```python
from build123d import *

# Parameters (mm, degrees)
SKETCH1_W           = 35
SKETCH1_H           = 30
BOSS_EXTRUDE5_DEPTH = 2
BOSS_EXTRUDE6_DEPTH = 1


with BuildPart() as part:
    # Sketch1 → Boss-Extrude5 (new body)
    with BuildSketch(Plane.XY):
        with Locations((0, -15)):
            Rectangle(SKETCH1_W, SKETCH1_H)
    extrude(amount=BOSS_EXTRUDE5_DEPTH)

    # Sketch1<7> → Boss-Extrude6 (add)
    with BuildSketch(Plane.XY):
        Polygon((-12.5, 10), (-12.5, 30), (-17.5, 30), (-17.5, 10), (-17.5, 0), (17.5, 0), (17.5, 10), (17.5, 30), (12.5, 30), (12.5, 10), (7.5, 10), (7.5, 30), (2.5, 30), (2.5, 10), (-2.5, 10), (-2.5, 30), (-7.5, 30), (-7.5, 10), align=None)
    extrude(amount=BOSS_EXTRUDE6_DEPTH)


solid = part.part
```
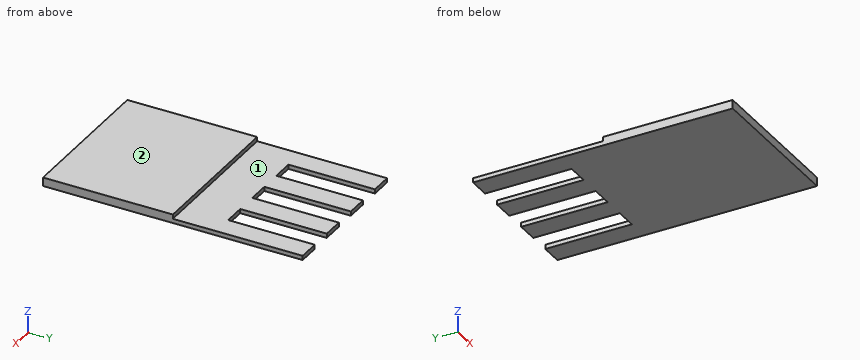
Verification items for the finished model (mm, model axes). Face numbers are marked on the shaded views. A direction names the side the tool comes from. Coordinates: 2 decimals unless noted, no trailing zeros. Loops run counter-clockwise (first coordinate to the right, second up) from the corner with the lowest first, then second, coordinate; pieces in that order, holes last. Notation, with made-up numbers: (-33.75, 79.25) - (-0.75, 79.25) arc R28 cw to (-0.75, 110.25) - close; hole circle Ø6 at (-35, 29.5). An arc over 180 degrees is marked (long way). Put each result on its own line as item: value.
Item 1: Section check C-C (z = 0.3). Enter the section's corners in (x, y).
Conclusion:
outline: (-17.5, -30) - (17.5, -30) - (17.5, 30) - (12.5, 30) - (12.5, 10) - (7.5, 10) - (7.5, 30) - (2.5, 30) - (2.5, 10) - (-2.5, 10) - (-2.5, 30) - (-7.5, 30) - (-7.5, 10) - (-12.5, 10) - (-12.5, 30) - (-17.5, 30) - close
Item 2: Gauge pin test, flat ends, axial feed: pin 1 Ø1 at (x, y) = (13.5, 2) entering from +Z; pin 2 Ø1.1 at (x, z) = (11, 0.5) entering from +Y. Record the tip position at first contact, or that the pin passes through.
Conclusion:
pin 1: stops at z = 1
pin 2: stops at y = 10
Item 3: Section check A-A (y = 21). Enter the section's corners in (x, z).
Conclusion:
outline: (-17.5, 0) - (-12.5, 0) - (-12.5, 1) - (-17.5, 1) - close; (-7.5, 0) - (-2.5, 0) - (-2.5, 1) - (-7.5, 1) - close; (2.5, 0) - (7.5, 0) - (7.5, 1) - (2.5, 1) - close; (12.5, 0) - (17.5, 0) - (17.5, 1) - (12.5, 1) - close
Item 4: Section check B-B (x = -11.5). Enter the section's corners in (y, z).
Conclusion:
outline: (-30, 0) - (10, 0) - (10, 1) - (0, 1) - (0, 2) - (-30, 2) - close
Item 5: Scan lines: line 1 along X through (y, z) = (19, 0.85); line 2 along Y through (x, z) = (-15.5, 1.65); line 3 along Z through (x, y) = (-1, 2.5). Record each from-to range of solid material in increasing order.
Conclusion:
line 1: x = -17.5 to -12.5, -7.5 to -2.5, 2.5 to 7.5, 12.5 to 17.5
line 2: y = -30 to 0
line 3: z = 0 to 1
Item 6: Set-up check for the marked faces 1 and 2: record each of +Z, -Z, +X, -X, +Y, -Y from which the full face is reachable in a straight line by a thin tool's end or side.
Conclusion:
face 1: +Z, +X, -X, +Y
face 2: +Z, +X, -X, +Y, -Y
